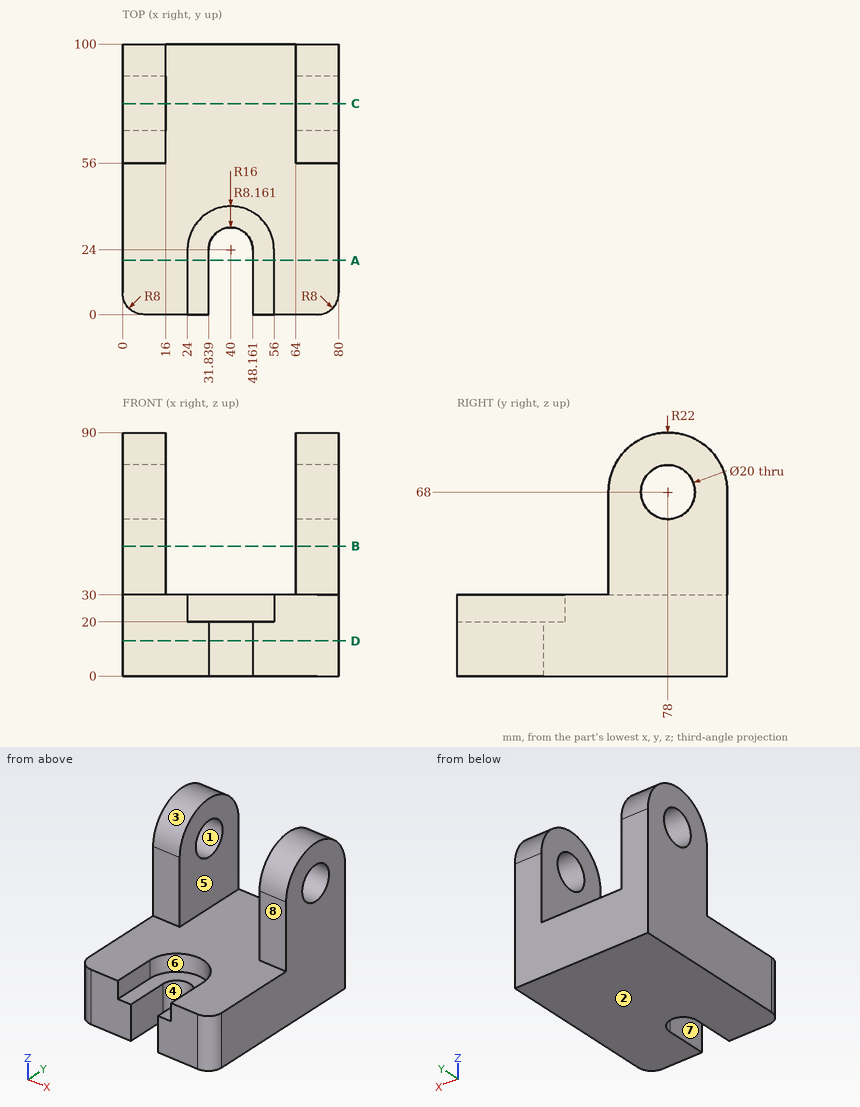
The drawing under review shows one solid part. Ordinate dimensions are in mm from its lowest x, y, z. A direction names the side the tool comes from. Coordinates: 2 decimals unless noted, no trailing zeros. Order: outer loops, then holes, each group sorted by start corner. A loop starts at its lowest first (then second) coordinate and runs counter-clockwise, first axis right, second up. Notation, with made-up numbers: M 7.25,-38.75 L 27.25,-38.75 A20 ccw 27.25,-20.75 Z; hole C -24,-5.5 d2. An arc over 180 degrees is marked long. Use a Markdown table: item, result.
(1) For the marked faces 5, 6, 7 and 8, list the 3-axis set-ups (+Z, -Z, +X, -X, +Y, -Y) from which the entire face can be reached by the end or side of a thin tool; tool diameter is ignored.
Worked answers:
| item | result |
|---|---|
| face 5 | +Z, +Y, -Y |
| face 6 | +Z, -Y |
| face 7 | +Z, -Z, -Y |
| face 8 | +Z, +X, -X, -Y |
(2) Add section C-C (y = 78). Give the boundary of the cut face in (x, z), then the cut area to 3 significant figures.
Worked answers:
| item | result |
|---|---|
| outline | M 0,0 L 80,0 L 80,58 L 64,58 L 64,30 L 16,30 L 16,58 L 0,58 Z; M 0,78 L 16,78 L 16,90 L 0,90 Z; M 64,78 L 80,78 L 80,90 L 64,90 Z |
| area | 3,680 mm2 |
(3) Add section B-B (z = 48). Give the boundary of the cut face in (x, y).
Worked answers:
| item | result |
|---|---|
| outline | M 0,56 L 16,56 L 16,100 L 0,100 Z; M 64,56 L 80,56 L 80,100 L 64,100 Z |
(4) Add section A-A (y = 20). Give the boundary of the cut face in (x, z), then the cut area to 3 significant figures.
Worked answers:
| item | result |
|---|---|
| outline | M 0,0 L 31.84,0 L 31.84,20 L 24,20 L 24,30 L 0,30 Z; M 48.16,0 L 80,0 L 80,30 L 56,30 L 56,20 L 48.16,20 Z |
| area | 1,750 mm2 |
(5) Draft analysis for pull direction Z (two halves, no side actions). For the marked faces 1, 2, 3 and 4, state which applies: released by +Z, released by -Z, zero draft, split by the parting line, or undercut.
Worked answers:
| item | result |
|---|---|
| face 1 | undercut |
| face 2 | released by -Z |
| face 3 | released by +Z |
| face 4 | zero draft |
(6) Wall thickness on probe 1 along Z at (x, y) = (8.5, 78); probe 2 along Y at (x, z) = (10.5, 68); probe 3 along X at (y, z) = (67, 46.5): over which ranges is each line inside the solid? List them lowest first.
Worked answers:
| item | result |
|---|---|
| probe 1 | z = 0 to 58, 78 to 90 |
| probe 2 | y = 56 to 68, 88 to 100 |
| probe 3 | x = 0 to 16, 64 to 80 |
(7) Add section D-D (z = 13). Give the boundary of the cut face in (x, y), then the cut area to 3 significant figures.
Worked answers:
| item | result |
|---|---|
| outline | M 0,8 A8 ccw 8,0 L 31.84,0 L 31.84,24 A8.16 cw 48.16,24 L 48.16,0 L 72,0 A8 ccw 80,8 L 80,100 L 0,100 Z |
| area | 7,480 mm2 |
(8) For P1, Ø10, axis at x = 17.5, y = 40, coming from the +Z side; P2, Ø13, axis at x = 4.5, z = 44.5, coming from the -Y side, all flat-tipped, find the tip position at first contact; note any pin that passes through.
Worked answers:
| item | result |
|---|---|
| P1 | stops at z = 30 |
| P2 | stops at y = 56 |
